The listing builds one solid part. Answer for the finished solid, in the listing's coordinates (mm). A direction names the side the tool comes from. Round coordinates to 2 decimals unless told otherwise and drop trailing zeros. Loops run counter-clockwise (first coordinate to the right, second up) from the corner with the lowest first, then second, coordinate; pieces in that order, holes last. Notation, with made-up numbers: (-1, -2) - (12, -2) arc R32 ccw to (12, 24) - close; hole circle Ø6 at (19.25, 39.5). An arc over 180 degrees is marked (long way). Write item = value, one per line. Start each with the question number.
1) Straight lines are drawn through the part: line 1 along Z through (x, y) = (0, -18.9); line 2 along X through (y, z) = (-18, -5); line 3 along Z through (x, y) = (-9.5, 18). For each, find the intervals that lie inside material, in ascending order.
2) A tool of negligible diameter and unlimited length cuts with its end or side. For faces 1 (the cylindrical face through (-1.08, -4.88, 39.86)), 2 (the flat face through (-2.2, -15, -1.6)), 3 (the cylindrical face through (0.81, -17.46, -1.34)), 4 (the flat face through (5, 17, -3)), from which of +Z, -Z, +X, -X, +Y, -Y can it reach the whole face along a straight path? Write none if from no direction.
3) Section B-B, the plane z = 38.5 is taken. Determine the outline of the cut face in (x, y).
4) Given pin 1 Ø19.5 at (x, y) = (-5.5, 0) entering from -Z; pin 2 Ø1.5 at (y, z) = (-18.5, -2) entering from +X; pin 3 Ø12 at (x, z) = (0, -5) entering from -Y; pin 4 Ø12 at (x, z) = (8.5, 2) entering from -Y, each flat-ended and moving along its own axis, determine where each tip first touches the part or whether it passes through.
5) For a pull along X with two mould halves and no side action, classify faces 5 (the flat face through (2, 5, 0)), 6 (the flat face through (5, -18, -3)), 7 (the cylindrical face through (-3, 18, -9)) as released by +X, released by -X, zero draft, split by the parting line, or undercut.
6) Section C-C, the plane z = 15.5 is taken. Determine the outline of the cut face in (x, y).
from build123d import *

# Parameters (mm, degrees)
SKETCH1_R           = 25
BOSS_EXTRUDE1_DEPTH = 30
SKETCH2_R           = 10
BOSS_EXTRUDE2_DEPTH = 20
SKETCH3_R           = 7.5
CUT_EXTRUDE1_DEPTH  = 20
SKETCH4_R           = 5
BOSS_EXTRUDE3_DEPTH = 20
BOSS_EXTRUDE4_START = 5
SKETCH5_R           = 10
BOSS_EXTRUDE4_DEPTH = 5
SKETCH7_W           = 10
SKETCH7_H           = 5
BOSS_EXTRUDE5_DEPTH = 10
SKETCH8_R           = 3.75
CUT_EXTRUDE2_DEPTH  = 5
CUT_EXTRUDE3_START  = -5
SKETCH9_R           = 3.75
CUT_EXTRUDE3_DEPTH  = 5
FILLET1_R           = 5
FILLET2_R           = 5
CUT_EXTRUDE4_START  = -15
SKETCH10_R          = 10
SKETCH10_R_2        = 7.5
CUT_EXTRUDE4_DEPTH  = 15
CUT_EXTRUDE5_START  = -5
SKETCH11_R          = 7.5
CUT_EXTRUDE5_DEPTH  = 5
BOSS_EXTRUDE6_START = 20
SKETCH12_R          = 5
BOSS_EXTRUDE6_DEPTH = 20


# Some blends are built 0.0001 mm under size
with BuildPart() as part:
    # Sketch1 → Boss-Extrude1 (new body)
    with BuildSketch(Plane.XY):
        Circle(SKETCH1_R)
    extrude(amount=BOSS_EXTRUDE1_DEPTH)

    # Sketch2 → Boss-Extrude2 (add)
    with BuildSketch(Plane.XY.offset(30)):
        Circle(SKETCH2_R)
    extrude(amount=BOSS_EXTRUDE2_DEPTH)

    # Sketch3 → Cut-Extrude1 (cut)
    with BuildSketch(Plane.XY.offset(50)):
        Circle(SKETCH3_R)
    extrude(amount=-CUT_EXTRUDE1_DEPTH, mode=Mode.SUBTRACT)

    # Sketch4 → Boss-Extrude3 (add)
    with BuildSketch(Plane.XY.offset(30)):
        Circle(SKETCH4_R)
    extrude(amount=BOSS_EXTRUDE3_DEPTH)

    # Sketch5 → Boss-Extrude4 (add)
    with BuildSketch(Plane(origin=(0, 0, 0), x_dir=(-1, 0, 0), z_dir=(0, 0, -1)).offset(BOSS_EXTRUDE4_START)):
        with Locations(Location((0, 0, 0), (0, 0, 180))):
            Circle(SKETCH5_R)
    extrude(amount=-BOSS_EXTRUDE4_DEPTH)

    # Sketch7 → Boss-Extrude5 (add)
    with BuildSketch(Plane(origin=(0, 0, 0), x_dir=(-1, 0, 0), z_dir=(0, 0, -1))):
        with Locations((0, 17.5)):
            Rectangle(SKETCH7_W, SKETCH7_H)
        with Locations((0, -17.5)):
            Rectangle(SKETCH7_W, SKETCH7_H)
    extrude(amount=BOSS_EXTRUDE5_DEPTH)

    # Sketch8 → Cut-Extrude2 (cut)
    with BuildSketch(Plane(origin=(0, 20, 0), x_dir=(1, 0, 0), z_dir=(0, 1, 0))):
        with Locations(Location((0, 5, 0), (0, 0, 180))):
            Circle(SKETCH8_R)
    extrude(amount=-CUT_EXTRUDE2_DEPTH, mode=Mode.SUBTRACT)

    # Sketch9 → Cut-Extrude3 (cut)
    with BuildSketch(Plane(origin=(0, -20, 0), x_dir=(-1, 0, 0), z_dir=(0, -1, 0)).offset(CUT_EXTRUDE3_START)):
        with Locations((0, 5)):
            Circle(SKETCH9_R)
    extrude(amount=CUT_EXTRUDE3_DEPTH, mode=Mode.SUBTRACT)

    # Fillet1
    # the kernel refuses this fillet: 5 mm, written as the material it takes off along each edge
    with BuildSketch(Plane(origin=(0, 0, 30), x_dir=(1, 0, 0), z_dir=(0, -1, 0))) as fillet1_piece_1:
        with BuildLine():
            CenterArc((25 - FILLET1_R, -FILLET1_R), FILLET1_R, 0, 90)
            Line((25 - FILLET1_R, 0), (25, 0))
            Line((25, 0), (25, -FILLET1_R))
        make_face()
    revolve(axis=Axis((0, 0, 30), (0, 0, 1)), mode=Mode.SUBTRACT)
    with BuildSketch(Plane(origin=(0, 0, 0), x_dir=(1, 0, 0), z_dir=(0, -1, 0))) as fillet1_piece_2_section:
        with BuildLine():
            CenterArc((25 - FILLET1_R, FILLET1_R), FILLET1_R, 270, 90)
            Line((25 - FILLET1_R, 0), (25, 0))
            Line((25, 0), (25, FILLET1_R))
        make_face()
    fillet1_piece_2 = revolve(axis=Axis((0, 0, 0), (0, 0, 1)), mode=Mode.PRIVATE)
    fillet1_piece_2 = split(fillet1_piece_2, bisect_by=Plane(origin=(5, 14.511659558, 1.419610571), z_dir=(1, 0, 0)), keep=Keep.TOP, mode=Mode.PRIVATE)
    add(fillet1_piece_2, mode=Mode.SUBTRACT)
    with BuildSketch(Plane(origin=(0, 0, 0), x_dir=(1, 0, 0), z_dir=(0, -1, 0))) as fillet1_piece_3_section:
        with BuildLine():
            CenterArc((25 - FILLET1_R, FILLET1_R), FILLET1_R, 270, 90)
            Line((25 - FILLET1_R, 0), (25, 0))
            Line((25, 0), (25, FILLET1_R))
        make_face()
    fillet1_piece_3 = revolve(axis=Axis((0, 0, 0), (0, 0, 1)), mode=Mode.PRIVATE)
    fillet1_piece_3 = split(fillet1_piece_3, bisect_by=Plane(origin=(4.6e-08, 20, 1.116734198), z_dir=(0, 1, 0)), keep=Keep.TOP, mode=Mode.PRIVATE)
    add(fillet1_piece_3, mode=Mode.SUBTRACT)
    with BuildSketch(Plane(origin=(0, 0, 0), x_dir=(1, 0, 0), z_dir=(0, -1, 0))) as fillet1_piece_4_section:
        with BuildLine():
            CenterArc((25 - FILLET1_R, FILLET1_R), FILLET1_R, 270, 90)
            Line((25 - FILLET1_R, 0), (25, 0))
            Line((25, 0), (25, FILLET1_R))
        make_face()
    fillet1_piece_4 = revolve(axis=Axis((0, 0, 0), (0, 0, 1)), mode=Mode.PRIVATE)
    fillet1_piece_4 = split(fillet1_piece_4, bisect_by=Plane(origin=(-4.6e-08, -20, 1.116734198), z_dir=(0, -1, 0)), keep=Keep.TOP, mode=Mode.PRIVATE)
    add(fillet1_piece_4, mode=Mode.SUBTRACT)
    with BuildSketch(Plane(origin=(0, 0, 0), x_dir=(1, 0, 0), z_dir=(0, -1, 0))) as fillet1_piece_5_section:
        with BuildLine():
            CenterArc((25 - FILLET1_R, FILLET1_R), FILLET1_R, 270, 90)
            Line((25 - FILLET1_R, 0), (25, 0))
            Line((25, 0), (25, FILLET1_R))
        make_face()
    fillet1_piece_5 = revolve(axis=Axis((0, 0, 0), (0, 0, 1)), mode=Mode.PRIVATE)
    fillet1_piece_5 = split(fillet1_piece_5, bisect_by=Plane(origin=(-5, 0, 1.419610538), z_dir=(-1, 0, 0)), keep=Keep.TOP, mode=Mode.PRIVATE)
    add(fillet1_piece_5, mode=Mode.SUBTRACT)

    # Fillet2
    fillet2_edges = [part.edges().sort_by_distance(p)[0] for p in [
        (5, -17.5, -10),
        (-5, -17.5, -10),
        (5, 17.5, -10),
        (-5, 17.5, -10),
    ]]
    fillet(fillet2_edges, radius=FILLET2_R - 0.0001)  # a hair under: the kernel refuses the full size

    # Sketch10 → Cut-Extrude4 (cut)
    with BuildSketch(Plane.XY.offset(50).offset(CUT_EXTRUDE4_START)):
        Circle(SKETCH10_R)
        Circle(SKETCH10_R_2, mode=Mode.SUBTRACT)
    extrude(amount=CUT_EXTRUDE4_DEPTH, mode=Mode.SUBTRACT)

    # Sketch11 → Cut-Extrude5 (cut)
    with BuildSketch(Plane(origin=(0, 0, -5), x_dir=(-1, 0, 0), z_dir=(0, 0, -1)).offset(CUT_EXTRUDE5_START)):
        with Locations(Location((0, 0, 0), (0, 0, 180))):
            Circle(SKETCH11_R)
    extrude(amount=CUT_EXTRUDE5_DEPTH, mode=Mode.SUBTRACT)

    # Sketch12 → Boss-Extrude6 (add)
    with BuildSketch(Plane(origin=(0, 0, 0), x_dir=(-1, 0, 0), z_dir=(0, 0, -1)).offset(BOSS_EXTRUDE6_START)):
        with Locations(Location((0, 0, 0), (0, 0, 180))):
            Circle(SKETCH12_R)
    extrude(amount=-BOSS_EXTRUDE6_DEPTH)


solid = part.part
Geometry check:
q1.line_1 = -10 to -8.75, -1.25 to 30
q1.line_2 = -5 to -3.75, 3.75 to 5
q1.line_3 = 0.01 to 29.99
q2.face_1 = +Z
q2.face_2 = -Z, +X, -X
q2.face_3 = -Y
q2.face_4 = -Z, +X, +Y
q3.outline = circle Ø10 at (0, 0)
q4.pin_1 = -20
q4.pin_2 = 5
q4.pin_3 = -23
q4.pin_4 = -24.79
q5.face_5 = undercut
q5.face_6 = released by +X
q5.face_7 = released by -X
q6.outline = circle Ø50 at (0, 0)
